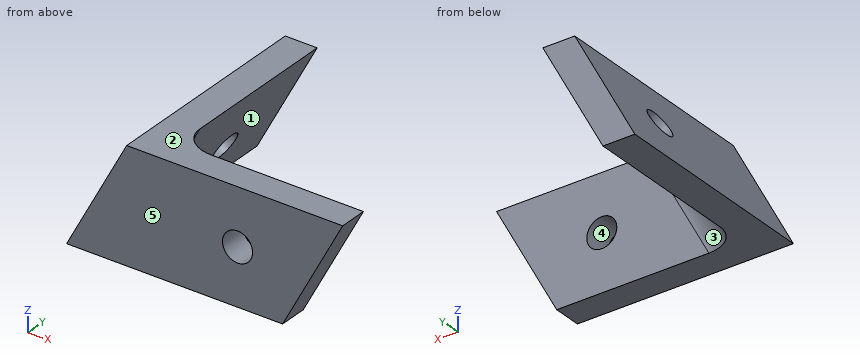
```python
from build123d import *

# Parameters (mm, degrees)
EXTRUDE_1_DEPTH     = 3
EXTRUDE_2_DEPTH     = 20
CUT_EXTRUDE_1_REACH = 86.581
SKETCH_3_R          = 1.6
CUT_EXTRUDE_2_REACH = 57.839
SKETCH_4_R          = 1.6
FILLET_1_R          = 3


with BuildPart() as part:
    # 草图1 → 凸台-拉伸1 (new body)
    with BuildSketch(Plane(origin=(0, 0, 0), x_dir=(1, 0, 0), z_dir=(0, 1, 0))):
        Polygon((-80, 15), (-57, 15), (-50.6, 3), (-73.6, 3), align=None)
    extrude(amount=EXTRUDE_1_DEPTH)

    # 草图2 → 凸台-拉伸2 (add)
    with BuildSketch(Plane(origin=(0, 3, 0), x_dir=(1, 0, 0), z_dir=(0, 1, 0))):
        Polygon((-80, 15), (-73.6, 3), (-70.2, 3), (-76.6, 15), align=None)
    extrude(amount=EXTRUDE_2_DEPTH)

    # 草图3 → 切除-拉伸1 (cut, up to next)
    with BuildSketch(Plane(origin=(0, 0, 0), x_dir=(1, 0, 0), z_dir=(0, 1, 0)), mode=Mode.PRIVATE) as cut_extrude_1_sk1:
        with Locations(Location((-61.8, 9, 0), (0, 0, 270))):
            Circle(SKETCH_3_R)
    cut_extrude_1_tool1 = extrude(cut_extrude_1_sk1.sketch, amount=CUT_EXTRUDE_1_REACH, mode=Mode.PRIVATE) & part.part
    add(cut_extrude_1_tool1.solids().sort_by_distance((-61.8, 0, -9))[0], mode=Mode.SUBTRACT)

    # 草图4 → 切除-拉伸2 (cut, up to next)
    with BuildSketch(Plane(origin=(-56.055363322, 0, 29.896193772), x_dir=(-0.4705882352941182, 0, -0.8823529411764703), z_dir=(0.8823529411764703, 0, -0.4705882352941182)), mode=Mode.PRIVATE) as cut_extrude_2_sk1:
        with Locations(Location((44.082352941, 15, 0), (0, 0, 180))):
            Circle(SKETCH_4_R)
    cut_extrude_2_tool1 = extrude(cut_extrude_2_sk1.sketch, amount=CUT_EXTRUDE_2_REACH, mode=Mode.PRIVATE) & part.part
    add(cut_extrude_2_tool1.solids().sort_by_distance((-76.8, 15, -9))[0], mode=Mode.SUBTRACT)

    # 圆角1
    fillet_1_edges = [part.edges().sort_by_distance(p)[0] for p in [
        (-73.4, 3, -9),
    ]]
    fillet(fillet_1_edges, radius=FILLET_1_R)


solid = part.part
```
Check sheet for the modelled part. Datum: model origin and axes. Units: mm. Face numbers are marked on the shaded views. A direction names the side the tool comes from. Round coordinates to 2 decimals unless told otherwise and drop trailing zeros. Order: outer loops, then holes, each group sorted by start corner. A loop starts at its lowest first (then second) coordinate and runs counter-clockwise, first axis right, second up. Notation, with made-up numbers: (64.5, 84.25) - (108.5, 84.25) arc R33 cw to (108.5, 120.25) - close; hole circle Ø1 at (-8, 77). An arc over 180 degrees is marked (long way). Answer as CSV lines item,"result". Start each with the question number.
1) Tool access check on the marked faces 1 and 2. Record the directions out of +Z, -Z, +X, -X, +Y, -Y that give a thin tool (end or side, any length) a straight path to the whole face; none if there is none.
2) Section check D-D (z = -10.25). Give the number of separate pieces and of enclosed holes in the cut face, then the cut area to 3 significant figures.
3) Draft check along X on the marked faces 3, 4 and 5. Enter one of: +X half, -X half, draft (parallel to the pull), parting line (faces both ways), or undercut.
4) Section check A-A (x = -61.8). Record the cut outline in (y, z), then the cut area to 3 significant figures.
5) Scan lines: probe 1 along Z at (x, y) = (-61.8, 1.95); probe 2 along X at (y, z) = (2, -9); probe 3 along Y at (x, z) = (-59.5, -7.5). Record each from-to range of solid material in increasing order.
6) Section check C-C (y = 2). Record the cut outline in (x, z).
7) Depth check by flat-ended pin: pin 1 (4 mm diameter, centred on y = 13, z = -10, fed in from +X); pin 2 (2 mm diameter, centred on y = 20, z = -4.5, fed in from +X); pin 3 (1.5 mm diameter, centred on x = -70.5, z = -9.5, fed in from +Y). Enter the tip coordinate at first touch or a pass-through.
8) Section check B-B (y = 15.75). Record the cut outline in (x, z), then the cut area to 3 significant figures.
Determined:
1,face 1,"-Z, +X, +Y"
1,face 2,"+Z, +X, -X, +Y, -Y"
2,separate pieces,"3"
2,enclosed holes,"0"
2,area,"124 mm^2"
3,face 3,"+X half"
3,face 4,"undercut"
3,face 5,"draft"
4,outline,"(0, -15) - (3, -15) - (3, -10.6) - (0, -10.6) - close; (0, -7.4) - (3, -7.4) - (3, -3) - (0, -3) - close"
4,area,"26.4 mm^2"
5,probe 1,"-15 to -10.6, -7.4 to -3"
5,probe 2,"-76.8 to -63.4, -60.2 to -53.8"
5,probe 3,"0 to 3"
6,outline,"(-80, -15) - (-57, -15) - (-50.6, -3) - (-73.6, -3) - close; hole circle Ø3.2 at (-61.8, -9)"
7,pin 1,"x = -72.87"
7,pin 2,"x = -70.47"
7,pin 3,"y = 3.16"
8,outline,"(-80, -15) - (-76.6, -15) - (-74.82, -11.66) - (-77.47, -10.25) - close; (-76.13, -7.75) - (-73.49, -9.16) - (-70.2, -3) - (-73.6, -3) - close"
8,area,"32.3 mm^2"
